```python
from build123d import *
from build123d.topology import SkipClean

# Parameters (mm, degrees)
SKETCH_7_R               = 12.6
CUT_EXTRUDE_1_DEPTH      = 15
SKETCH_8_R               = 16.5
CUT_EXTRUDE_2_DEPTH      = 1
CUT_EXTRUDE_3_DEPTH      = 25
PATTERN_CIRCULAR_1_COUNT = 4
SKETCH_12_R              = 16.5
SKETCH_12_R_2            = 12.6
EXTRUDE_1_DEPTH          = 1
CUT_EXTRUDE_4_DEPTH      = 15
PATTERN_CIRCULAR_2_COUNT = 4


with BuildPart() as part:
    # Эскиз2 → Повернуть1 (revolve)
    with BuildSketch(Plane.XY):
        with BuildLine():
            Line((0, 0), (0, 28.5))
            add(Edge.make_bspline(
                [(0, 28.5), (31.309007967, 24.448027272), (52.310724818, 0)],
                knots=[0, 0, 0, 1, 1, 1], degree=2))
            Line((52.310724818, 0), (28.5, 0))
            Line((28.5, 0), (0, 0))
        make_face()
    revolve(axis=Axis((-1000, 0, 0), (1, 0, 0)))

    # Эскиз7 → Вырез-Вытянуть1 (cut)
    with BuildSketch(Plane.ZY):
        Circle(SKETCH_7_R)
    extrude(amount=-CUT_EXTRUDE_1_DEPTH, mode=Mode.SUBTRACT)

    # Эскиз8 → Вырез-Вытянуть2 (cut)
    with BuildSketch(Plane.ZY):
        Circle(SKETCH_8_R)
    extrude(amount=-CUT_EXTRUDE_2_DEPTH, mode=Mode.SUBTRACT)

    # Эскиз11 → Вырез-Вытянуть3 (cut)
    with BuildSketch(Plane.ZY):
        with BuildLine():
            Line((-9.747574085, 26.781239692), (-7.695453225, 21.143083968))
            Line((-7.695453225, 21.143083968), (-5.643332365, 15.504928243))
            ThreePointArc((-5.643332365, 15.504928243), (0, 16.5), (5.643332365, 15.504928243))
            Line((5.643332365, 15.504928243), (7.695453225, 21.143083968))
            Line((7.695453225, 21.143083968), (9.747574085, 26.781239692))
            ThreePointArc((9.747574085, 26.781239692), (0, 28.5), (-9.747574085, 26.781239692))
        make_face()
    cut_extrude_3 = extrude(amount=-CUT_EXTRUDE_3_DEPTH, mode=Mode.SUBTRACT)

    # Круговой массив1: Вырез-Вытянуть3 ×4 about axis
    pattern_circular_1_axis = Axis((1, 0, 0), (-1, 0, 0))
    for i in range(1, PATTERN_CIRCULAR_1_COUNT):
        add(cut_extrude_3.rotate(pattern_circular_1_axis, i * 360 / PATTERN_CIRCULAR_1_COUNT), mode=Mode.SUBTRACT)

    # Эскиз12 → Бобышка-Вытянуть1 (add)
    with SkipClean():  # the faces are left unmerged after this step: merging them gives an invalid solid
        with BuildSketch(Plane.ZY.offset(-1)):
            Circle(SKETCH_12_R)
            Circle(SKETCH_12_R_2, mode=Mode.SUBTRACT)
        extrude(amount=EXTRUDE_1_DEPTH)

    # Эскиз13 → Вырез-Вытянуть4 (cut)
    with SkipClean():  # the faces are left unmerged after this step: merging them gives an invalid solid
        with BuildSketch(Plane.ZY):
            with BuildLine():
                Line((-14.006579324, 17.608683529), (-10.271491505, 12.913034588))
                ThreePointArc((-10.271491505, 12.913034588), (0, 16.5), (10.271491505, 12.913034588))
                Line((10.271491505, 12.913034588), (14.006579324, 17.608683529))
                ThreePointArc((14.006579324, 17.608683529), (0, 22.5), (-14.006579324, 17.608683529))
            make_face()
        cut_extrude_4 = extrude(amount=-CUT_EXTRUDE_4_DEPTH, mode=Mode.SUBTRACT)

    # Круговой массив2: Вырез-Вытянуть4 ×4 about axis
    with SkipClean():  # the faces are left unmerged after this step: merging them gives an invalid solid
        pattern_circular_2_axis = Axis((0, 0, 0), (-1, 0, 0))
        for i in range(1, PATTERN_CIRCULAR_2_COUNT):
            add(cut_extrude_4.rotate(pattern_circular_2_axis, i * 360 / PATTERN_CIRCULAR_2_COUNT), mode=Mode.SUBTRACT)


solid = part.part
```
The model under review builds one solid part; all positions refer to its coordinate system, in mm. A direction names the side the tool comes from. Give positions to 0.01 mm unless a question says otherwise; leave off trailing zeros. Write item = value, one per line. Start each with the question number.
Q1. Clearance check with flat-ended pins moving along their axes: pin 1 (4 mm diameter, centred on y = 17.5, z = -9.5, fed in from -X); pin 2 (12 mm diameter, centred on y = 5.5, z = -5.5, fed in from +X); pin 3 (12 mm diameter, centred on x = 32, y = 13.5, fed in from -Z); pin 4 (2.5 mm diameter, centred on y = -12, z = -15, fed in from -X). State where each tip first meets the part, or that it passes through.
Q2. For line 1 (Z direction, x = 35.5, y = 8); line 2 (Y direction, x = 8.5, z = -22); line 3 (Z direction, x = 22, y = -5), list the stretches that pass through material, from the lowest coordinate up.
Q3. Machinability: for faces 3 (the face through (25, 18, 0)), 4 (the face through (15, -10, -17)), 5 (the face through (25, 0, -19)), which of the approach directions +Z, -Z, +X, -X, +Y, -Y give a long, thin tool a straight path to every point of the face, cutting with its end or side? Answer none if there is none.
Q4. Mouldability with a two-part tool opening along Z and no side actions: class faces 1 (the face through (7.395, -12.165, -15.294)), 2 (the face through (25, 0, 19)) as released by +Z, released by -Z, zero draft, split by the parting line, or undercut.
Result set:
q1.pin_1 = 15
q1.pin_2 = 50.75
q1.pin_3 = -17.59
q1.pin_4 = 0
q2.line_1 = -12.93 to 12.93
q2.line_2 = -15.62 to -8.01, 8.01 to 15.62
q2.line_3 = -15.72 to 15.72
q3.face_3 = -X, +Y
q3.face_4 = -X
q3.face_5 = -Z, -X
q4.face_1 = undercut
q4.face_2 = zero draft
